Geometry: final body of the model. Coordinates: model frame, mm. Face numbers are marked on the shaded views. A direction names the side the tool comes from. Round coordinates to 2 decimals unless told otherwise and drop trailing zeros. Write each loop counter-clockwise with the first axis right and the second up, starting at its lowest first coordinate (ties: lowest second). Pieces come first, ordered by that corner, then holes. Notation, with made-up numbers: (23, 16) -> (76, 16) arc R20 cw to (76, 27) -> close; hole circle Ø3 at (-26, 89.5). An arc over 180 degrees is marked (long way). Use one line per item in the form item = value. Start each with the question number.
1. Line query: L1, parallel to X at y = 0, z = 0.35; L2, parallel to X at y = 0, z = 0.8; L3, parallel to Z at x = 84, y = 9. Output: solid intervals per line, ascending.
2. Reachability of the marked faces 1 and 2 from +Z, -Z, +X, -X, +Y, -Y: full face, straight path, thin tool, end or side. Return the list, or none.
3. Cut plane C-C, the plane z = 7. Return the cut outline in (x, y).
4. Pin query (flat end, axial travel): pin 1 Ø7 at (x, y) = (47.5, -3) entering from +Z; pin 2 Ø5 at (y, z) = (8, 6) entering from -X; pin 3 Ø8 at (y, z) = (5, 15) entering from -X. Return the tip coordinate at first contact, or that it passes through.
```python
from build123d import *

# Parameters (mm, degrees)
BOSS_EXTRUDE1_DEPTH     = 1.524
FILLET1_R               = 1.524
SKETCH3_R               = 6.35
BOSS_EXTRUDE3_DEPTH     = 25.4
CUT_EXTRUDE4_DEPTH      = 97.813899613
CUT_EXTRUDE4_DEPTH_BACK = 97.813899613
SKETCH5_R               = 6.35


with BuildPart() as part:
    # Sketch2 → Boss-Extrude1 (new, symmetric)
    with BuildSketch(Plane.XY):
        with BuildLine():
            Line((0, 13.135315222), (79.359196135, 13.135315222))
            ThreePointArc((79.359196135, 13.135315222), (92.494511357, 0), (79.359196135, -13.135315222))
            Line((79.359196135, -13.135315222), (0, -13.135315222))
            ThreePointArc((0, -13.135315222), (-13.135315222, 0), (0, 13.135315222))
        make_face()
    extrude(amount=BOSS_EXTRUDE1_DEPTH, both=True)

    # Fillet1
    fillet1_edges = [part.edges().sort_by_distance(p)[0] for p in [
        (92.494511357, 0, -1.524),
        (39.679598067, -13.135315222, -1.524),
        (-13.135315222, 0, -1.524),
        (92.494511357, 0, 1.524),
        (39.679598067, -13.135315222, 1.524),
        (-13.135315222, 0, 1.524),
        (39.679598067, 13.135315222, -1.524),
        (39.679598067, 13.135315222, 1.524),
    ]]
    fillet(fillet1_edges, radius=FILLET1_R - 0.0001)  # a hair under: the kernel refuses the full size

    # Sketch3 → Boss-Extrude3 (add)
    with BuildSketch(Plane.XY):
        Circle(SKETCH3_R)
    extrude(amount=BOSS_EXTRUDE3_DEPTH)

    # Sketch5 → Cut-Extrude4 (cut, two sides: drawn at the far end of the back side and taken through both)
    with BuildSketch(Plane.XY.offset(-CUT_EXTRUDE4_DEPTH_BACK)):
        with Locations((79.359196135, 0)):
            Circle(SKETCH5_R)
    extrude(amount=CUT_EXTRUDE4_DEPTH + CUT_EXTRUDE4_DEPTH_BACK, mode=Mode.SUBTRACT)


solid = part.part
```
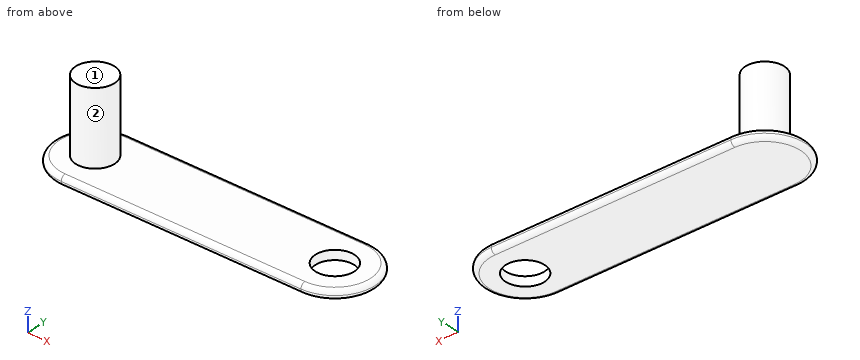
Outcome:
q1.L1 = -13.09 to 73.01, 85.71 to 92.45
q1.L2 = -12.91 to 73.01, 85.71 to 92.27
q1.L3 = -1.52 to 1.52
q2.face_1 = +Z, +X, -X, +Y, -Y
q2.face_2 = +Z
q3.outline = circle Ø12.7 at (0, 0)
q4.pin_1 = 1.52
q4.pin_2 = -3.17
q4.pin_3 = -6.27
